The model under review builds one solid part; all positions refer to its coordinate system, in mm. Round coordinates to 2 decimals unless told otherwise and drop trailing zeros. Write each loop counter-clockwise with the first axis right and the second up, starting at its lowest first coordinate (ties: lowest second). Pieces come first, ordered by that corner, then holes.
Item 1: Add section B-B (z = -10.5). Give the boundary of the cut face in (x, y), plus the area to 3 significant figures.
Item 2: Add section A-A (z = -6). Give the boundary of the cut face in (x, y), plus the area to 3 significant figures.
Item 3: To check wall thickness, follow L1, parallel to Z at x = -14, y = 5; L2, parallel to Z at x = 7, y = 1.5; L3, parallel to Y at x = 0, z = -17.5. State the ranges of each line that lie inside material, in increasing order.
Item 4: Draft analysis for pull direction Y (two halves, no side actions). For faces 1 (the face through (0, 0, 0)), 2 (the face through (0, 0, 1)), 3 (the face through (-14.735, -4.64, -12.181)), state which applies: +Y half, -Y half, draft (parallel to the pull), parting line (faces both ways), or undercut.
Item 5: Clearance check with flat-ended pins moving along their axes: pin 1 Ø6 at (y, z) = (9.5, -16.5) entering from +X; pin 2 Ø8 at (x, y) = (-2.5, 0) entering from -Z; pin 3 Ø8 at (x, z) = (2, -11.5) entering from -Y; pin 4 Ø6 at (x, y) = (10.5, 3.5) entering from -Z. State where each tip first meets the part, or that it passes through.
```python
from build123d import *

# Parameters (mm, degrees)
F2_SIZE = 0.5


with BuildPart() as f1:
    # F0 (on Front) → F1 (revolve)
    with BuildSketch(Plane.XZ):
        with BuildLine():
            Line((-12.959872, 0), (0, 0))
            Line((0, 0), (0, 1))
            Line((0, 1), (-15.071469, 1))
            Line((-15.071469, 1), (-15.814245, -24.997144))
            Line((-15.814245, -24.997144), (-14.799996, -24.997144))
            Line((-14.799996, -24.997144), (-14.799996, -34.997144))
            Line((-14.799996, -34.997144), (-13.75, -35))
            Line((-13.75, -35), (-13.75, -0.790128))
            ThreePointArc((-13.75, -0.790128), (-13.518577, -0.231423), (-12.959872, 0))
        make_face()
    revolve(axis=Axis((0, 0, 35.289533), (0, 0, 1)))

    # F2
    f2_edges = [f1.edges().sort_by_distance(p)[0] for p in [
        (14.799996, 0, -34.997144),
    ]]
    chamfer(f2_edges, length=F2_SIZE)


solid = f1.part
```
Numbers:
1. outline: circle Ø30.8 at (0, 0); hole circle Ø27.5 at (0, 0)
1. area: 151 mm2
2. outline: circle Ø30.54 at (0, 0); hole circle Ø27.5 at (0, 0)
2. area: 139 mm2
3. L1: z = -25 to 1
3. L2: z = 0 to 1
3. L3: y = -15.6 to -13.75, 13.75 to 15.6
4. face 1: undercut
4. face 2: draft
4. face 3: parting line
5. pin 1: stops at x = 14.15
5. pin 2: stops at z = 0
5. pin 3: stops at y = -15.53
5. pin 4: stops at z = -35
